from build123d import *

# Parameters (mm, degrees)
F2_DEPTH  = 32.3
F3_DEPTH  = 32.3
F4_W      = 60.45
F4_H      = 21.25
F5_DEPTH  = 17.8
F0_R      = 1.625
F7_DEPTH  = 2.5
F8_DEPTH  = 125
F9_DEPTH  = 25
F10_DEPTH = 2.5


with BuildPart() as f2:
    # F1 (on Right) → F2 (new body)
    with BuildSketch(Plane.YZ):
        Polygon((-30.3661038332, 12.7279220614), (-17.6381817718, 0), (23, 0), (0, 22), (-12.7279220614, 34.7279220614), align=None)
    extrude(amount=F2_DEPTH)

    # F3 (add): a face of the model
    f3_faces = [f2.faces().sort_by_distance(p)[0] for p in [
        (0, -7.2105643806, 12.6516732047),
    ]]
    extrude(f3_faces, amount=F3_DEPTH)

    # F4 (on face) → F5 (cut)
    with BuildSketch(Plane(origin=(0, -24.6962676026, 19.7998753209), x_dir=(1, 0, 0), z_dir=(0, -0.780207847, 0.6255203557))):
        with Locations((0, 5.0346157827)):
            Rectangle(F4_W, F4_H)
    extrude(amount=-F5_DEPTH, mode=Mode.SUBTRACT)

    # F0 (on Top) → F7 (join)
    with BuildSketch(Plane.XY):
        with BuildLine():
            ThreePointArc((-18.8683877308, 14.6094391689), (-15.8539987253, 15.2350988211), (-14.5, 18))
            ThreePointArc((-14.5, 18), (-14.5324686308, 18.4756324252), (-14.6292721165, 18.9424402026))
            ThreePointArc((-14.6292721165, 18.9424402026), (-20.5018295404, 20.4476210799), (-18.8683877308, 14.6094391689))
        make_face()
        with Locations((-18, 18)):
            Circle(F0_R, mode=Mode.SUBTRACT)
        with BuildLine():
            ThreePointArc((-14.6292721165, 18.9424402026), (-14.5324686308, 18.4756324252), (-14.5, 18))
            ThreePointArc((-14.5, 18), (-15.8539987253, 15.2350988211), (-18.8683877308, 14.6094391689))
            ThreePointArc((-18.8683877308, 14.6094391689), (-12.4958401108, 0.0286551223), (-18.7836705303, -14.5888622866))
            ThreePointArc((-18.7836705303, -14.5888622866), (-15.8197301608, -15.26204028), (-14.5, -18))
            ThreePointArc((-14.5, -18), (-14.5324686308, -18.4756324252), (-14.6292721165, -18.9424402026))
            ThreePointArc((-14.6292721165, -18.9424402026), (-0.0113565012, -12.5687447065), (14.6204813838, -18.9104141492))
            ThreePointArc((14.6204813838, -18.9104141492), (15.4793732037, -15.5717412507), (18.7836705303, -14.5888622866))
            ThreePointArc((18.7836705303, -14.5888622866), (12.4958401108, 0.0286551223), (18.8683877308, 14.6094391689))
            ThreePointArc((18.8683877308, 14.6094391689), (15.5098110461, 15.5405368525), (14.6204813838, 18.9104141492))
            ThreePointArc((14.6204813838, 18.9104141492), (-0.0113565012, 12.5687447065), (-14.6292721165, 18.9424402026))
        make_face()
        with BuildLine():
            ThreePointArc((21.5, 18), (18.459175807, 21.4697489215), (14.6204813838, 18.9104141492))
            ThreePointArc((14.6204813838, 18.9104141492), (15.5098110461, 15.5405368525), (18.8683877308, 14.6094391689))
            ThreePointArc((18.8683877308, 14.6094391689), (20.7649011789, 15.8539987253), (21.5, 18))
        make_face()
        with Locations((18, 18)):
            Circle(F0_R, mode=Mode.SUBTRACT)
        with BuildLine():
            ThreePointArc((-14.5, -18), (-15.8197301608, -15.26204028), (-18.7836705303, -14.5888622866))
            ThreePointArc((-18.7836705303, -14.5888622866), (-20.532118995, -20.4162726243), (-14.6292721165, -18.9424402026))
            ThreePointArc((-14.6292721165, -18.9424402026), (-14.5324686308, -18.4756324252), (-14.5, -18))
        make_face()
        with Locations((-18, -18)):
            Circle(F0_R, mode=Mode.SUBTRACT)
        with BuildLine():
            ThreePointArc((21.5, -18), (20.73795972, -15.8197301608), (18.7836705303, -14.5888622866))
            ThreePointArc((18.7836705303, -14.5888622866), (15.4793732037, -15.5717412507), (14.6204813838, -18.9104141492))
            ThreePointArc((14.6204813838, -18.9104141492), (18.459175807, -21.4697489215), (21.5, -18))
        make_face()
        with Locations((18, -18)):
            Circle(F0_R, mode=Mode.SUBTRACT)
    extrude(amount=-F7_DEPTH)

    # F6 (on face) → F8 (cut)
    with BuildSketch(Plane.YZ.offset(32.3)):
        with BuildLine():
            Line((23, 0), (1.3185644747, 20.7387644155))
            ThreePointArc((1.3185644747, 20.7387644155), (7.8131331228, 8.5369425815), (18.6844021082, 0))
            Line((18.6844021082, 0), (23, 0))
        make_face()
    extrude(amount=-F8_DEPTH, mode=Mode.SUBTRACT)

    # F9 (cut): a face of the model
    f9_faces = [f2.faces().sort_by_distance(p)[0] for p in [
        (0.0105418264, 16.2029444185, 0),
    ]]
    extrude(f9_faces, amount=-F9_DEPTH, mode=Mode.SUBTRACT)

    # F10 (add, through all): faces of the model
    f10_faces = [f2.faces().sort_by_distance(p)[0] for p in [
        (23.7244305893, 0.3347471948, 0),
        (-23.7244305893, 0.3347471948, 0),
        (0.0105418264, -15.5866223713, 0),
    ]]
    extrude(f10_faces, amount=F10_DEPTH)


solid = f2.part
Read the model definition and answer for the solid it produces. Units are mm, in the model's axes. A direction names the side the tool comes from. Give positions to 0.01 mm unless a question says otherwise; leave off trailing zeros. Write each loop counter-clockwise with the first axis right and the second up, starting at its lowest first coordinate (ties: lowest second). Pieces come first, ordered by that corner, then holes. Notation, with made-up numbers: (-12.75, -27.75) - (34.25, -27.75) arc R12 cw to (34.25, -4.75) - close; hole circle Ø2 at (-16, -27.5). An arc over 180 degrees is marked (long way). Answer in a Markdown table with one row per item. Add a question column.
Item 1: Determine the mould class of faces 5 (the face through (-32.3, -6, 12)), 6 (the face through (0.22, 12.57, 0.03)), 7 (the face through (-30.225, -15, 18)) for opening direction Y: pulls with the +Y half, pulls with the -Y half, needs draft (parallel to the pull), parting line crosses it, or undercut.
Item 2: A tool of negligible diameter and unlimited length cuts with its end or side. For faces 1 (the face through (-0.423, -7.566, 12.71)), 2 (the face through (-18, 18, 0)), 3 (the face through (-27, 18.684, -1)), 4 (the face through (27, -17.638, -1)), from which of +Z, -Z, +X, -X, +Y, -Y can it reach the whole face along a straight path? Write none if from no direction.
Item 3: Section A-A, the plane x = 18 is taken. Write down the section's boundary in (y, z) (3 decimals), and give its area (3 significant figures).
Item 4: Section D-D, the plane y = 15.5 is taken. Write down the section's boundary in (x, z), and give its area (3 significant figures).
Item 5: Section B-B, the plane y = -6 is taken. Write down the section's boundary in (x, z) (1 decimal).
Item 6: Flat-ended cylindrical pins translate along their axes: P1, Ø2, axis at x = -22.5, z = 28, coming from the +Y side; P2, Ø1.3, axis at x = -29, z = -1, coming from the +Y side; P3, Ø3, axis at x = -17, y = 20, coming from the +Z side. Find the tip coordinate at first contact, or state that the pin passes through.
Item 7: Find the intervals of material crossed by L1, parallel to Y at x = -18, z = -1.6 (3 decimals); L2, parallel to X at y = -21.5, z = 15 (3 decimals); L3, parallel to X at y = -18, z = -1 (3 decimals), in increasing order.
Item 8: Section C-C, the plane z = 7 is taken. Write down the section's boundary in (x, y) (3 decimals), and give its area (3 significant figures).
Recorded:
| question | item | result |
|---|---|---|
| 1 | face 5 | needs draft |
| 1 | face 6 | pulls with the +Y half |
| 1 | face 7 | undercut |
| 2 | face 1 | none |
| 2 | face 2 | -Z |
| 2 | face 3 | +Z, -Z, -X, +Y |
| 2 | face 4 | -Z, +X, -Y |
| 3 | outline | (-30.366, 12.728) - (-17.638, 0) - (-16.375, 0) - (-16.375, -2.5) - (16.375, -2.5) - (16.375, 0) - (18.684, 0) arc R33.47 cw to (1.319, 20.739) - (0, 22) - (-12.728, 34.728) - (-14.901, 32.018) - (-1.013, 20.883) - (-14.305, 4.304) - (-28.193, 15.438) - close; (-21.5, -2.5) - (-19.625, -2.5) - (-19.625, 0) - (-21.5, 0) - close; (19.625, -2.5) - (21.5, -2.5) - (21.5, 0) - (19.625, 0) - close |
| 3 | area | 568 mm2 |
| 4 | outline | (-32.3, -2.5) - (-10.41, -2.5) - (-10.41, 1.79) - (-32.3, 1.79) - close; (10.43, -2.5) - (32.3, -2.5) - (32.3, 1.79) - (10.43, 1.79) - close |
| 4 | area | 188 mm2 |
| 5 | outline | (-32.3, -2.5) - (32.3, -2.5) - (32.3, 28) - (-32.3, 28) - close; hole (-30.2, 14.7) - (30.2, 14.7) - (30.2, 24.9) - (-30.2, 24.9) - close |
| 6 | P1 | stops at y = -5 |
| 6 | P2 | stops at y = 18.68 |
| 6 | P3 | stops at z = 0.09 |
| 7 | L1 | y = -21.5 to -19.625, -16.375 to 16.375, 19.625 to 21.5 |
| 7 | L2 | x = -32.3 to -30.225, 30.225 to 32.3 |
| 7 | L3 | x = -21.5 to -19.625, -16.375 to -13.692, 13.713 to 16.375, 19.625 to 21.5 |
| 8 | outline | (-32.3, -24.638) - (32.3, -24.638) - (32.3, 9.183) - (-32.3, 9.183) - close; hole (-30.225, -17.668) - (30.225, -17.668) - (30.225, -12.144) - (-30.225, -12.144) - close |
| 8 | area | 1,850 mm2 |
